Autodesk Fusion 360 part; units mm, degrees
sketch "Sketch1" plane through (0, 0, 0) normal (0, 0, 1) x (1, 0, 0)
  line L0 (0, 0) -> (-30, 0)
  line L1 (-30, 0) -> (-30, 15)
  line L2 (-30, 15) -> (0, 15)
  line L3 (0, 15) -> (0, 0)
  line L4 (-15, 0) -> (-15, 15)
  line L5 (-25, 10) -> (-20, 10)
  line L6 (-20, 10) -> (-20, 5)
  line L7 (-20, 5) -> (-25, 5)
  line L8 (-25, 5) -> (-25, 10)
  line L9 (-10, 10) -> (-5, 10)
  line L10 (-5, 10) -> (-5, 5)
  line L11 (-5, 5) -> (-10, 5)
  line L12 (-10, 5) -> (-10, 10)
  line L13 (-25.175, 10.175) -> (-19.825, 10.175)
  line L14 (-19.825, 10.175) -> (-19.825, 4.825)
  line L15 (-19.825, 4.825) -> (-25.175, 4.825)
  line L16 (-25.175, 4.825) -> (-25.175, 10.175)
  line L17 (-10.175, 10.175) -> (-4.825, 10.175)
  line L18 (-4.825, 10.175) -> (-4.825, 4.825)
  line L19 (-4.825, 4.825) -> (-10.175, 4.825)
  line L20 (-10.175, 4.825) -> (-10.175, 10.175)
  dimension "d1" = 30
  dimension "d2" = 15
  dimension "d7" = -0.175
  dimension "d8" = -0.175
extrude "Extrude1" add sketch "Sketch1" along normal blind 10 contours L0 L2 L3 L4 | L0 L1 L2 L4 | L13 L14 L15 L16 | L17 L18 L19 L20
extrude "Extrude2" add sketch "Sketch1" along normal blind 15 contours L5 L6 L7 L8 | L9 L10 L11 L12
extrude "Extrude3" cut sketch "Sketch1" along normal blind 5.175 contours L5 L6 L7 L8 | L9 L10 L11 L12 | L13 L14 L15 L16 | L17 L18 L19 L20
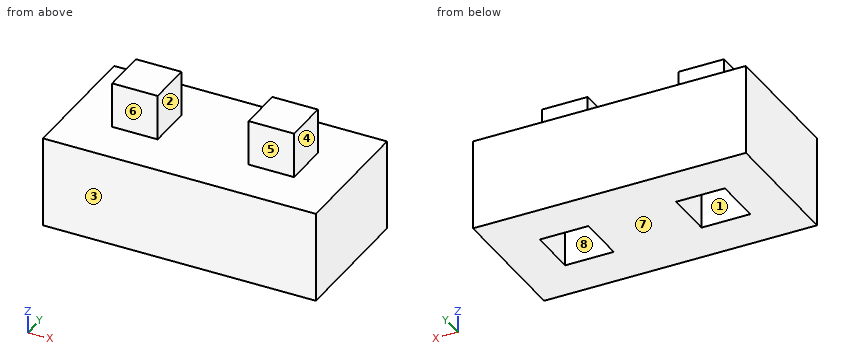
Here's how the part is built. I have some questions about the finished solid (model axes, mm). Face numbers are marked on the shaded views. A direction names the side the tool comes from. Give positions to 0.01 mm unless a question says otherwise; leave off trailing zeros. Write each loop counter-clockwise with the first axis right and the second up, starting at its lowest first coordinate (ties: lowest second). Pieces come first, ordered by that corner, then holes. Notation, with made-up numbers: (77.25, -9) -> (110.25, -9) arc R15 cw to (110.25, 15) -> close; hole circle Ø3 at (34, 23). An arc over 180 degrees is marked (long way). Use one line per item in the form item = value.
1) Suppose I cut it at C-C (z = 12). Please give me the cut outline in (x, y), and give its area (3 significant figures).
Verdict:
outline = (-25, 5) -> (-20, 5) -> (-20, 10) -> (-25, 10) -> close; (-10, 5) -> (-5, 5) -> (-5, 10) -> (-10, 10) -> close
area = 50.0 mm2
2) On a 3-axis mill with a long thin cutter (end or side, diameter ignored), from which of +Z, -Z, +X, -X, +Y, -Y can I reach the whole of each face in a straight line? I mean the marked faces 1, 2, 3, 4 and 5. Say none if no direction works.
Verdict:
face_1 = -Z
face_2 = +Z, +Y, -Y
face_3 = +Z, -Z, +X, -X, -Y
face_4 = +Z, +X, +Y, -Y
face_5 = +Z, +X, -X, -Y
3) Suppose I cut it at A-A (z = 1.25). Please give me the cut outline in (x, y) (3 decimals), and give its area (3 significant figures).
Verdict:
outline = (-30, 0) -> (0, 0) -> (0, 15) -> (-30, 15) -> close; hole (-25.175, 4.825) -> (-19.825, 4.825) -> (-19.825, 10.175) -> (-25.175, 10.175) -> close; hole (-10.175, 4.825) -> (-4.825, 4.825) -> (-4.825, 10.175) -> (-10.175, 10.175) -> close
area = 393 mm2
4) We'd pull the mould along Y, two halves only. Please class the marked faces 6, 7 and 8: +Y half, -Y half, draft (parallel to the pull), parting line (faces both ways), or undercut.
Verdict:
face_6 = -Y half
face_7 = draft
face_8 = undercut
5) I'm going to push flat-ended pins straight in: pin 1 (1.5 mm diameter, centred on x = -8, z = 13, fed in from +Y); pin 2 (3 mm diameter, centred on x = -23.5, y = 2, fed in from +Z); pin 3 (4 mm diameter, centred on x = -7, z = 13, fed in from -Y). Where does each tip first touch, or does it pass through?
Verdict:
pin_1 = 10
pin_2 = 10
pin_3 = 5
6) If I drill on L1, parallel to Y at x = -25, z = 3.25 (3 decimals); L2, parallel to Y at x = -5.25, z = 13.25; L3, parallel to Z at x = -3, y = 7, over which ranges is the centre line in solid material (lowest first)? Write a range as [from, to].
Verdict:
L1 = [0, 4.825], [10.175, 15]
L2 = [5, 10]
L3 = [0, 10]
7) Suppose I cut it at B-B (x = -8). Please give me the cut outline in (y, z) (3 decimals), and give its area (3 significant figures).
Verdict:
outline = (0, 0) -> (4.825, 0) -> (4.825, 5.175) -> (10.175, 5.175) -> (10.175, 0) -> (15, 0) -> (15, 10) -> (10, 10) -> (10, 15) -> (5, 15) -> (5, 10) -> (0, 10) -> close
area = 147 mm2
8) Suppose I cut it at D-D (y = 9.5). Please give me the cut outline in (x, z) (3 decimals).
Verdict:
outline = (-30, 0) -> (-25.175, 0) -> (-25.175, 5.175) -> (-19.825, 5.175) -> (-19.825, 0) -> (-10.175, 0) -> (-10.175, 5.175) -> (-4.825, 5.175) -> (-4.825, 0) -> (0, 0) -> (0, 10) -> (-5, 10) -> (-5, 15) -> (-10, 15) -> (-10, 10) -> (-20, 10) -> (-20, 15) -> (-25, 15) -> (-25, 10) -> (-30, 10) -> close
